Print and shaded views of the part. All mm, measured from the part's lowest x, y and z. A direction names the side the tool comes from. Give positions to 0.01 mm unless a question says otherwise; leave off trailing zeros. Order: outer loops, then holes, each group sorted by start corner. A loop starts at its lowest first (then second) coordinate and runs counter-clockwise, first axis right, second up. Notation, with made-up numbers: (-27, 8) -> (17, 8) arc R22 cw to (17, 20) -> close; hole circle Ø1 at (0, 78.5). An arc over 180 degrees is marked (long way). One line per question, with ' | ' between items. Start each with the question number.
(1) Cut at C-C (z = 57.5). Give the cut face in (x, y).
(2) Pull direction Z, two halves, no side cores. Call the marked faces 1, 2, 3 and 4: +Z half, -Z half, draft (parallel to the pull), parting line (faces both ways), or undercut.
(3) Drill centre lines: L1, parallel to Z at x = 203, y = 213; L2, parallel to Y at x = 191, z = 16; L3, parallel to X at y = 11, z = 81.5. Where is each one in solid material? Low to high. Write a range as from..to.
(4) Cut at D-D (x = 26.5). Give the cut face in (y, z).
(5) Pin check, flat tips, straight feed: pin 1 Ø10 at (x, z) = (179, 94.5) entering from -Y; pin 2 Ø19 at (x, z) = (148.5, 49) entering from +Y; pin 3 Ø10 at (y, z) = (95, 42.5) entering from +X. Stop position of each tip, or through.
(6) Which spindle directions (+Z, -Z, +X, -X, +Y, -Y) get a long thin tool onto all of the face, cutting with end or side? Do the marked faces 5, 6 and 7. Say none if no direction does.
(7) Cut at B-B (z = 40). Give the cut face in (x, y).
(8) Cut at A-A (x = 203.2). Give the cut face in (y, z).
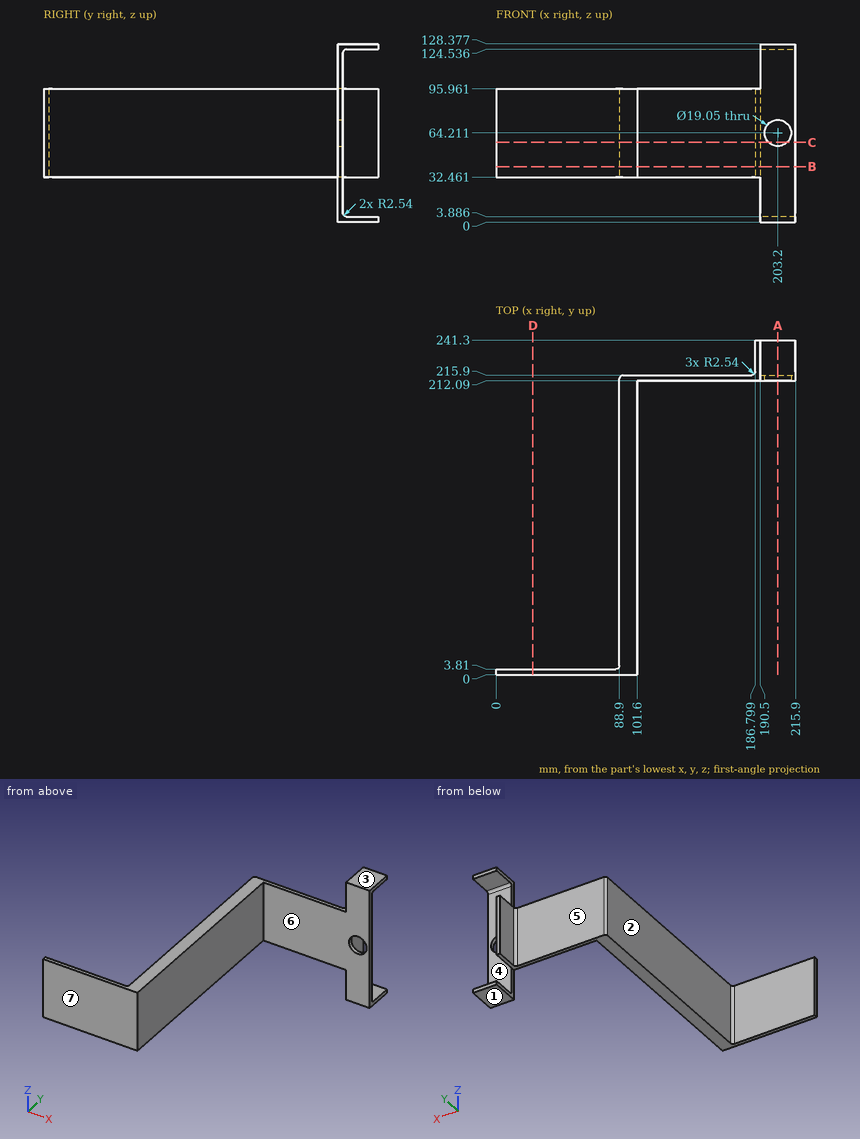
Result set:
1) outline: (0, 0) -> (101.6, 0) -> (101.6, 212.09) -> (196.44, 212.09) -> (196.44, 215.9) -> (190.5, 215.9) -> (190.5, 241.3) -> (186.8, 241.3) -> (186.8, 218.44) arc R2.54 cw to (184.26, 215.9) -> (91.44, 215.9) arc R2.54 ccw to (88.9, 213.36) -> (88.9, 6.35) arc R2.54 cw to (86.36, 3.81) -> (0, 3.81) -> close; (209.96, 212.09) -> (215.9, 212.09) -> (215.9, 215.9) -> (209.96, 215.9) -> close
2) face 1: -Z half | face 2: draft | face 3: +Z half | face 4: undercut
3) L1: z = 0..54.69, 73.73..128.38 | L2: y = 212.09..215.9 | L3: x = 88.9..101.6
4) outline: (0, 32.46) -> (3.81, 32.46) -> (3.81, 95.96) -> (0, 95.96) -> close
5) pin 1: stops at y = 212.09 | pin 2: stops at y = 215.9 | pin 3: stops at x = 101.6
6) face 5: +Z, -Z, -X, +Y | face 6: +Z, -Z, +X, -Y | face 7: +Z, -Z, +X, -X, -Y
7) outline: (0, 0) -> (101.6, 0) -> (101.6, 212.09) -> (215.9, 212.09) -> (215.9, 215.9) -> (190.5, 215.9) -> (190.5, 241.3) -> (186.8, 241.3) -> (186.8, 218.44) arc R2.54 cw to (184.26, 215.9) -> (91.44, 215.9) arc R2.54 ccw to (88.9, 213.36) -> (88.9, 6.35) arc R2.54 cw to (86.36, 3.81) -> (0, 3.81) -> close
8) outline: (212.09, 0) -> (241.3, 0) -> (241.3, 3.89) -> (218.44, 3.89) arc R2.54 cw to (215.9, 6.43) -> (215.9, 54.69) -> (212.09, 54.69) -> close; (212.09, 73.74) -> (215.9, 73.74) -> (215.9, 122) arc R2.54 cw to (218.44, 124.54) -> (241.3, 124.54) -> (241.3, 128.38) -> (212.09, 128.38) -> close
